Work out the finished part from the listing and answer in its coordinate system (mm). A direction names the side the tool comes from. Coordinates: 2 decimals unless noted, no trailing zeros. Order: outer loops, then holes, each group sorted by start corner. A loop starts at its lowest first (then second) coordinate and runs counter-clockwise, first axis right, second up. Notation, with made-up numbers: M 13.5,-28 L 34.5,-28 A24 ccw 34.5,8 Z; hole C 16,46.25 d9. An arc over 180 degrees is marked long. Answer in a Markdown table with one row per item. Add a question column.
Item 1: Which of the six approach directions +Z, -Z, +X, -X, +Y, -Y give full straight-line access (tool end or side, diameter ignored) to faces 1 (the face through (97.644, -7.455, -11.135)), 2 (the face through (-329.702, -14.997, -11.135)), 3 (the face through (7, 34.925, 0))?
Item 2: Consider line 1 (Z direction, x = 182, y = -27) (3 decimals); line 2 (Y direction, x = -73, z = 2.25) (3 decimals); line 3 (Y direction, x = -342.9, z = -11). Determine where each line is inside the solid, lowest interval first. Write a range as from..to.
Item 3: The mould has two halves that part along Y. Classify faces 4 (the face through (-6, -38.1, 0)), 5 (the face through (100.026, -12.072, 11.09)), 6 (the face through (504.825, 14, -10)): released by +Y, released by -Y, zero draft, split by the parting line, or undercut.
Item 4: Flat-ended cylindrical pins translate along their axes: pin 1 Ø4 at (x, z) = (396.875, 0) entering from -Y; pin 2 Ø3 at (x, z) = (-73.025, 0) entering from +Y (3 decimals); pin 3 Ø3 at (x, z) = (339.725, 0) entering from -Y (3 decimals). Find the tip coordinate at first contact, or state that the pin passes through.
Item 5: The part is cut by section A-A (x = -114.3). Write down the section's boundary in (y, z) (1 decimal).
from build123d import *

# Parameters (mm, degrees)
SKETCH1_W                                           = 1009.65
SKETCH1_H                                           = 76.2
SKETCH1_R                                           = 14.2875
BOSS_EXTRUDE2_DEPTH                                 = 12.7
SKETCH3_W                                           = 19.05
SKETCH3_H                                           = 69.85
CUT_EXTRUDE2_DEPTH                                  = 1011.448426442
CUT_EXTRUDE3_DEPTH                                  = 507.897475457
FILLET1_R                                           = 12.7
SKETCH9_R                                           = 1.7272
CUT_EXTRUDE4_DEPTH                                  = 2.54
SKETCH12_R                                          = 1.7272
CUT_EXTRUDE7_DEPTH                                  = 5.08
CSK_FOR_1_4_FLAT_HEAD_MACHINE_SCREW_100_D           = 6.7564
CSK_FOR_1_4_FLAT_HEAD_MACHINE_SCREW_100_CSINK_D     = 12.8778
CSK_FOR_1_4_FLAT_HEAD_MACHINE_SCREW_100_CSINK_ANGLE = 100
CUT_EXTRUDE8_START                                  = -6.35
SKETCH17_R                                          = 1.7272
CUT_EXTRUDE8_DEPTH                                  = 6.35
SKETCH18_R                                          = 17.4625
CUT_EXTRUDE9_DEPTH                                  = 3.81
F_1_4_0_25_DIAMETER_HOLE1_D                         = 6.35
F_10_32_TAPPED_HOLE1_D                              = 4.0386
F_10_32_TAPPED_HOLE1_DEPTH                          = 13.716
F_10_32_TAPPED_HOLE1_TIP                            = 1.213317848


with BuildPart() as part:
    # Sketch1 → Boss-Extrude2 (new, symmetric)
    with BuildSketch(Plane.XY):
        Rectangle(SKETCH1_W, SKETCH1_H)
        with Locations((-114.3, -12.7)):
            Circle(SKETCH1_R, mode=Mode.SUBTRACT)
        with Locations((114.3, -12.7)):
            Circle(SKETCH1_R, mode=Mode.SUBTRACT)
        with Locations((-342.9, -9.525)):
            Circle(SKETCH1_R, mode=Mode.SUBTRACT)
        with Locations((342.9, -9.525)):
            Circle(SKETCH1_R, mode=Mode.SUBTRACT)
    extrude(amount=BOSS_EXTRUDE2_DEPTH, both=True)

    # Sketch3 → Cut-Extrude2 (cut, through all)
    with BuildSketch(Plane(origin=(504.825, 0, 0), x_dir=(0, 0, -1), z_dir=(1, 0, 0))):
        Rectangle(SKETCH3_W, SKETCH3_H)
    extrude(amount=-CUT_EXTRUDE2_DEPTH, mode=Mode.SUBTRACT)

    # Sketch4 → Cut-Extrude3 (cut, through all)
    with BuildSketch(Plane.XY.offset(12.7)):
        Polygon((-504.825, -38.1), (-504.825, -19.05), (-428.625, -38.1), align=None)
        Polygon((428.625, -38.1), (504.825, -38.1), (504.825, -19.05), align=None)
    extrude(amount=-CUT_EXTRUDE3_DEPTH, mode=Mode.SUBTRACT)

    # Fillet1
    fillet1_edges = [part.edges().sort_by_distance(p)[0] for p in [
        (-504.825, -19.05, 11.1125),
        (-504.825, -19.05, -11.1125),
    ]]
    fillet(fillet1_edges, radius=FILLET1_R)

    # Sketch9 → Cut-Extrude4 (cut)
    with BuildSketch(Plane(origin=(0, 38.1, 0), x_dir=(1, 0, 0), z_dir=(0, 1, 0))):
        with Locations(Location((492.125, 0, 0), (0, 0, 270))):
            Circle(SKETCH9_R)
        with Locations(Location((479.425, 0, 0), (0, 0, 270))):
            Circle(SKETCH9_R)
        with Locations(Location((466.725, 0, 0), (0, 0, 270))):
            Circle(SKETCH9_R)
        with Locations(Location((454.025, 0, 0), (0, 0, 270))):
            Circle(SKETCH9_R)
        with Locations(Location((441.325, 0, 0), (0, 0, 270))):
            Circle(SKETCH9_R)
    extrude(amount=-CUT_EXTRUDE4_DEPTH, mode=Mode.SUBTRACT)

    # Sketch12 → Cut-Extrude7 (cut)
    with BuildSketch(Plane(origin=(0, 38.1, 0), x_dir=(1, 0, 0), z_dir=(0, 1, 0))):
        with Locations(Location((-98.425, 0, 0), (0, 0, 270))):
            Circle(SKETCH12_R)
        with Locations(Location((-85.725, 0, 0), (0, 0, 270))):
            Circle(SKETCH12_R)
        with Locations(Location((-73.025, 0, 0), (0, 0, 270))):
            Circle(SKETCH12_R)
        with Locations(Location((-60.325, 0, 0), (0, 0, 270))):
            Circle(SKETCH12_R)
        with Locations(Location((-47.625, 0, 0), (0, 0, 270))):
            Circle(SKETCH12_R)
        with Locations(Location((-34.925, 0, 0), (0, 0, 270))):
            Circle(SKETCH12_R)
        with Locations(Location((-22.225, 0, 0), (0, 0, 270))):
            Circle(SKETCH12_R)
    extrude(amount=-CUT_EXTRUDE7_DEPTH, mode=Mode.SUBTRACT)

    # CSK for 1/4 Flat Head Machine Screw (100)2 (through all)
    with Locations(Plane.XY.offset(12.7)):
        with Locations((66.675, -12.7), (161.925, -12.7)):
            CounterSinkHole(CSK_FOR_1_4_FLAT_HEAD_MACHINE_SCREW_100_D / 2, CSK_FOR_1_4_FLAT_HEAD_MACHINE_SCREW_100_CSINK_D / 2, counter_sink_angle=CSK_FOR_1_4_FLAT_HEAD_MACHINE_SCREW_100_CSINK_ANGLE)

    # Sketch17 → Cut-Extrude8 (cut)
    with BuildSketch(Plane(origin=(0, -38.1, 0), x_dir=(-1, 0, 0), z_dir=(0, -1, 0)).offset(CUT_EXTRUDE8_START)):
        with Locations(Location((-415.925, 0, 0), (0, 0, 90))):
            Circle(SKETCH17_R)
        with Locations(Location((-396.875, 0, 0), (0, 0, 90))):
            Circle(SKETCH17_R)
        with Locations(Location((-377.825, 0, 0), (0, 0, 90))):
            Circle(SKETCH17_R)
        with Locations(Location((-358.775, 0, 0), (0, 0, 90))):
            Circle(SKETCH17_R)
        with Locations(Location((-339.725, 0, 0), (0, 0, 90))):
            Circle(SKETCH17_R)
        with Locations(Location((-320.675, 0, 0), (0, 0, 90))):
            Circle(SKETCH17_R)
        with Locations(Location((-301.625, 0, 0), (0, 0, 90))):
            Circle(SKETCH17_R)
        with Locations(Location((-282.575, 0, 0), (0, 0, 90))):
            Circle(SKETCH17_R)
        with Locations(Location((-263.525, 0, 0), (0, 0, 90))):
            Circle(SKETCH17_R)
        with Locations(Location((-244.475, 0, 0), (0, 0, 90))):
            Circle(SKETCH17_R)
        with Locations(Location((-225.425, 0, 0), (0, 0, 90))):
            Circle(SKETCH17_R)
        with Locations(Location((-206.375, 0, 0), (0, 0, 90))):
            Circle(SKETCH17_R)
        with Locations(Location((-187.325, 0, 0), (0, 0, 90))):
            Circle(SKETCH17_R)
        with Locations(Location((-168.275, 0, 0), (0, 0, 90))):
            Circle(SKETCH17_R)
        with Locations(Location((-149.225, 0, 0), (0, 0, 90))):
            Circle(SKETCH17_R)
        with Locations(Location((-130.175, 0, 0), (0, 0, 90))):
            Circle(SKETCH17_R)
        with Locations(Location((-111.125, 0, 0), (0, 0, 90))):
            Circle(SKETCH17_R)
        with Locations(Location((-92.075, 0, 0), (0, 0, 90))):
            Circle(SKETCH17_R)
        with Locations(Location((-73.025, 0, 0), (0, 0, 90))):
            Circle(SKETCH17_R)
        with Locations(Location((-53.975, 0, 0), (0, 0, 90))):
            Circle(SKETCH17_R)
        with Locations(Location((-34.925, 0, 0), (0, 0, 90))):
            Circle(SKETCH17_R)
        with Locations(Location((-15.875, 0, 0), (0, 0, 90))):
            Circle(SKETCH17_R)
        with Locations(Location((3.175, 0, 0), (0, 0, 90))):
            Circle(SKETCH17_R)
        with Locations(Location((22.225, 0, 0), (0, 0, 270))):
            Circle(SKETCH17_R)
        with Locations(Location((41.275, 0, 0), (0, 0, 90))):
            Circle(SKETCH17_R)
        with Locations(Location((60.325, 0, 0), (0, 0, 270))):
            Circle(SKETCH17_R)
    extrude(amount=CUT_EXTRUDE8_DEPTH, mode=Mode.SUBTRACT)

    # Sketch18 → Cut-Extrude9 (cut)
    with BuildSketch(Plane(origin=(0, 0, -12.7), x_dir=(-1, 0, 0), z_dir=(0, 0, -1))):
        with Locations((-114.3, -12.7)):
            Circle(SKETCH18_R)
    extrude(amount=-CUT_EXTRUDE9_DEPTH, mode=Mode.SUBTRACT)

    # 1/4 (0.25) Diameter Hole1 (through all)
    with Locations(Plane.XY.offset(12.7)):
        with Locations((460.375, 25.4), (460.375, 0)):
            Hole(F_1_4_0_25_DIAMETER_HOLE1_D / 2)

    # #10-32 Tapped Hole1
    with Locations(Plane(origin=(0, 38.1, 0), x_dir=(1, 0, 0), z_dir=(0, 1, 0))):
        with Locations((-155.575, 0), (-200.025, 0)):
            Hole(F_10_32_TAPPED_HOLE1_D / 2, depth=F_10_32_TAPPED_HOLE1_DEPTH)
            with Locations((0, 0, -(F_10_32_TAPPED_HOLE1_DEPTH + F_10_32_TAPPED_HOLE1_TIP / 2))):  # 118° drill point
                Cone(0, F_10_32_TAPPED_HOLE1_D / 2, F_10_32_TAPPED_HOLE1_TIP, mode=Mode.SUBTRACT)


solid = part.part
Reply:
| question | item | result |
|---|---|---|
| 1 | face 1 | -Z |
| 1 | face 2 | +Z, -Z |
| 1 | face 3 | +X, -X |
| 2 | line 1 | z = -12.7..-9.525, 9.525..12.7 |
| 2 | line 2 | y = -38.1..-34.925, 34.925..38.1 |
| 2 | line 3 | y = -38.1..-23.81, 4.76..38.1 |
| 3 | face 4 | released by -Y |
| 3 | face 5 | undercut |
| 3 | face 6 | zero draft |
| 4 | pin 1 | stops at y = -38.1 |
| 4 | pin 2 | stops at y = -34.925 |
| 4 | pin 3 | stops at y = 34.925 |
| 5 | outline | M -38.1,-12.7 L -27,-12.7 L -27,-9.5 L -34.9,-9.5 L -34.9,9.5 L -27,9.5 L -27,12.7 L -38.1,12.7 Z; M 1.6,-12.7 L 38.1,-12.7 L 38.1,12.7 L 1.6,12.7 L 1.6,9.5 L 34.9,9.5 L 34.9,-9.5 L 1.6,-9.5 Z |
